Drawing for the job (mm, zero at the part's lowest x, y, z). Coordinates: 2 decimals unless noted, no trailing zeros. Loops run counter-clockwise (first coordinate to the right, second up) from the corner with the lowest first, then second, coordinate; pieces in that order, holes last. Notation, with made-up numbers: (43.5, 79) - (65.5, 79) arc R7 cw to (65.5, 87) - close; hole circle Ø11 at (19.5, 8.25). An arc over 180 degrees is marked (long way). One line per item, written item: value.
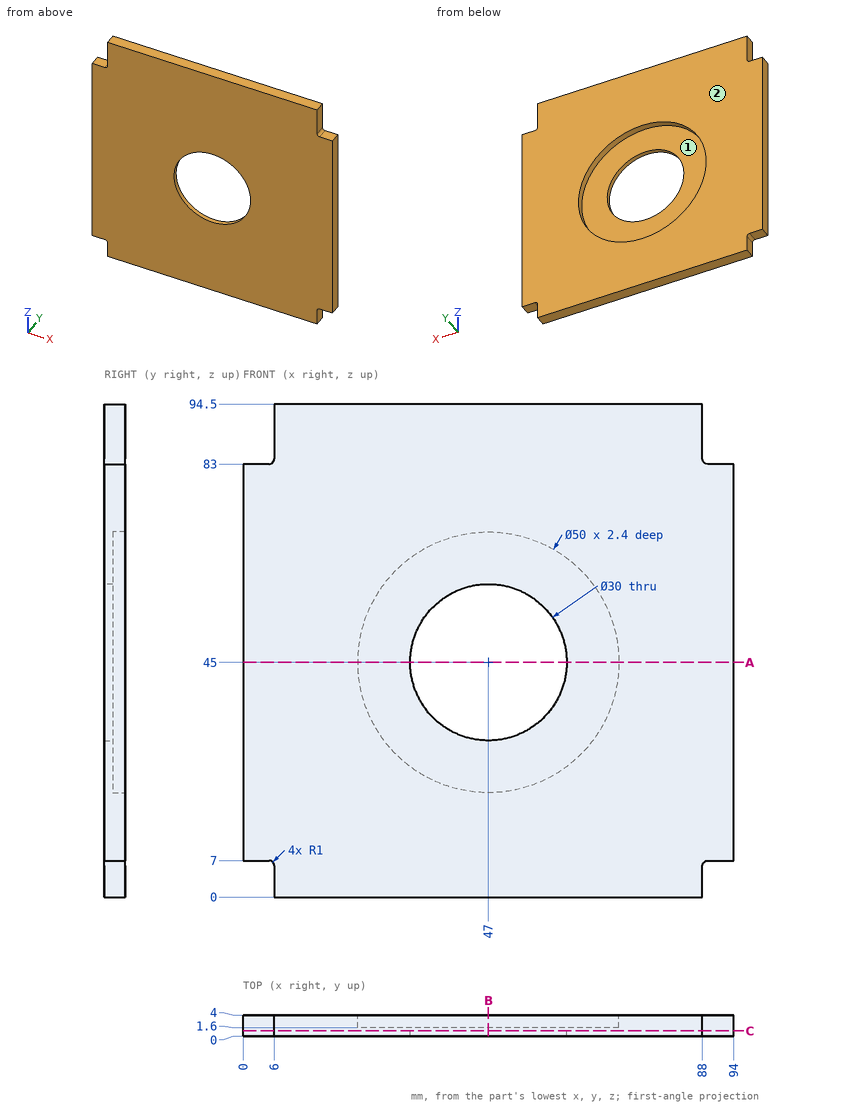
Item 1: Cut at C-C, the plane y = 1. Write the cut outline in (x, z), then the cut area to 4 significant figures.
Check result:
outline: (0, 7) - (5, 7) arc R1 cw to (6, 6) - (6, 0) - (88, 0) - (88, 6) arc R1 cw to (89, 7) - (94, 7) - (94, 83) - (89, 83) arc R1 cw to (88, 84) - (88, 94.5) - (6, 94.5) - (6, 84) arc R1 cw to (5, 83) - (0, 83) - close; hole circle Ø30 at (47, 45)
area: 7,955 mm^2
Item 2: Drop flat-ended pins along their axis: P1, Ø2, axis at x = 90.5, y = 2.5, coming from the +Z side; P2, Ø2, axis at x = 90.5, y = 3, coming from the -Z side; P3, Ø8, axis at x = 37.5, z = 44, coming from the -Y side; P4, Ø2, axis at y = 1.5, z = 3.5, coming from the -X side. Give the stop position or say it passes through.
Check result:
P1: stops at z = 83
P2: stops at z = 7
P3: passes through
P4: stops at x = 6
Item 3: Cut at A-A, the plane z = 45. Write the cut outline in (x, y).
Check result:
outline: (0, 0) - (32, 0) - (32, 1.6) - (22, 1.6) - (22, 4) - (0, 4) - close; (62, 0) - (94, 0) - (94, 4) - (72, 4) - (72, 1.6) - (62, 1.6) - close
Item 4: Cut at B-B, the plane x = 47. Write the cut outline in (y, z), then the cut area to 3 significant figures.
Check result:
outline: (0, 0) - (4, 0) - (4, 20) - (1.6, 20) - (1.6, 30) - (0, 30) - close; (0, 60) - (1.6, 60) - (1.6, 70) - (4, 70) - (4, 94.5) - (0, 94.5) - close
area: 210 mm^2
Item 5: Pull direction Z, two halves, no side cores. Call the marked faces 1 and 2: released by +Z, released by -Z, zero draft, split by the parting line, or undercut.
Check result:
face 1: undercut
face 2: zero draft
Item 6: Probe probe 1 along X at (y, z) = (2.45, 45); probe 2 along X at (y, z) = (0.55, 45); probe 3 along X at (y, z) = (1.7, 90.5). List the from-to ranges inside material, lowest first. Write a range as from..to.
Check result:
probe 1: x = 0..22, 72..94
probe 2: x = 0..32, 62..94
probe 3: x = 6..88
